Check sheet for the modelled part. Datum: model origin and axes. Units: mm. A direction names the side the tool comes from. Give positions to 0.01 mm unless a question says otherwise; leave off trailing zeros. Write each loop counter-clockwise with the first axis right and the second up, starting at its lowest first coordinate (ties: lowest second). Pieces come first, ordered by that corner, then holes. Notation, with made-up numbers: (-4, -16.5) - (5, -16.5) arc R12 cw to (5, 0.5) - close; hole circle Ø7 at (16, 82.25). An arc over 180 degrees is marked (long way). Return JSON: item names as keys, results as strings. Group by question number.
```python
from build123d import *

# Parameters (mm, degrees)
SKETCH_1_R           = 29
EXTRUDE_1_DEPTH      = 15
SKETCH_2_R           = 1.55
SKETCH_2_R_2         = 5.1
CUT_EXTRUDE_1_DEPTH  = 44.669211122
EXTRUDE_2_DEPTH      = 71
SKETCH_12_W          = 70
SKETCH_12_H          = 15
EXTRUDE_3_DEPTH      = 71
FILLET_5_R           = 10
SKETCH_22_W          = 71
SKETCH_22_H          = 103
CUT_EXTRUDE_11_DEPTH = 10
SKETCH_4_R           = 40
CUT_EXTRUDE_2_DEPTH  = 56
SKETCH_5_R           = 15.6
SKETCH_5_R_2         = 1.55
CUT_EXTRUDE_3_DEPTH  = 171.241005636
SKETCH_6_W           = 32.2
SKETCH_6_H           = 32.2
CUT_EXTRUDE_4_DEPTH  = 23.7
CUT_EXTRUDE_5_DEPTH  = 171.241005636
SKETCH_8_W           = 10
SKETCH_8_H           = 50
CUT_EXTRUDE_6_DEPTH  = 10
FILLET_1_R           = 10
FILLET_2_R           = 10
FILLET_3_R           = 10
SKETCH_17_R          = 22.5
CUT_EXTRUDE_7_DEPTH  = 7
SKETCH_18_R          = 24
CUT_EXTRUDE_8_DEPTH  = 0.5
EXTRUDE_START        = 10
SKETCH_19_R          = 15
SKETCH_19_R_2        = 1.55
SKETCH_19_R_3        = 5.1
EXTRUDE_5_DEPTH      = 10
SKETCH_20_R          = 3
CUT_EXTRUDE_9_DEPTH  = 3
SKETCH_23_R          = 1.5
CUT_EXTRUDE_12_DEPTH = 161.262160225
SKETCH_27_R          = 3
CUT_EXTRUDE_14_DEPTH = 3
SKETCH_28_W          = 10
SKETCH_28_H          = 6
EXTRUDE_6_DEPTH      = 5
FILLET_6_R           = 5
EXTRUDE_7_DEPTH      = 10
EXTRUDE_8_DEPTH      = 6


# Some blends are built 0.0001 mm under size
with BuildPart() as part:
    # Sketch 1 → Extrude 1 (new body)
    with BuildSketch(Plane.XY):
        Circle(SKETCH_1_R)
    extrude(amount=EXTRUDE_1_DEPTH)

    # Sketch 2 → Cut-Extrude 1 (cut, through all)
    with BuildSketch(Plane.XY.offset(15)):
        with Locations((-5.125, 8.876760389)):
            Circle(SKETCH_2_R)
        with Locations((5.125, 8.876760389)):
            Circle(SKETCH_2_R)
        with Locations((10.25, 0)):
            Circle(SKETCH_2_R)
        with Locations((5.125, -8.876760389)):
            Circle(SKETCH_2_R)
        Circle(SKETCH_2_R_2)
        with Locations((-5.125, -8.876760389)):
            Circle(SKETCH_2_R)
        with Locations((-10.25, 0)):
            Circle(SKETCH_2_R)
    extrude(amount=-CUT_EXTRUDE_1_DEPTH, mode=Mode.SUBTRACT)

    # Sketch 17 → Cut-Extrude 7 (cut)
    with BuildSketch(Plane.XY.offset(15)):
        Circle(SKETCH_17_R)
    extrude(amount=-CUT_EXTRUDE_7_DEPTH, mode=Mode.SUBTRACT)

    # Sketch 18 → Cut-Extrude 8 (cut)
    with BuildSketch(Plane.XY.offset(8)):
        Circle(SKETCH_18_R)
    extrude(amount=-CUT_EXTRUDE_8_DEPTH, mode=Mode.SUBTRACT)


with BuildPart() as body_2:
    # Sketch 3 → Extrude 2 (new body)
    with BuildSketch(Plane.XY):
        with BuildLine():
            ThreePointArc((-29, 0), (0, 29), (29, 0))
            Line((29, 0), (29, 95))
            Line((29, 95), (-9, 95))
            Line((-9, 95), (-9, 145))
            Line((-9, 145), (-29, 145))
            Line((-29, 145), (-29, 0))
        make_face()
    extrude(amount=EXTRUDE_2_DEPTH)

    # Sketch 12 → Extrude 3 (add)
    with BuildSketch(Plane.XY.offset(71)):
        with Locations((0, 34.5)):
            Rectangle(SKETCH_12_W, SKETCH_12_H)
    extrude(amount=-EXTRUDE_3_DEPTH)

    # Fillet 5
    # the kernel refuses this fillet: 10 mm, written as the material it takes off along each edge
    with BuildSketch(Plane(origin=(35, 42, 93.912878475), x_dir=(0, -1, 0), z_dir=(0, 0, -1))) as fillet_5_piece_1:
        with BuildLine():
            CenterArc((9.16515139, 10), FILLET_5_R, 203.578178478, 66.421821522)
            Line((0, 6), (-0.183303028, 5.92))
            ThreePointArc((-0.183303028, 5.92), (-0.2, 3), (-0.2, 0))
            Line((-0.2, 0), (0, -0.2))
            Line((0, -0.2), (9.16515139, -0.2))
            Line((9.16515139, -0.2), (9.16515139, 0))
        make_face()
    extrude(amount=116.82575695, mode=Mode.SUBTRACT)
    with BuildSketch(Plane(origin=(-35, 42, 93.912878475), x_dir=(0, -1, 0), z_dir=(0, 0, -1))) as fillet_5_piece_2:
        with BuildLine():
            CenterArc((9.16515139, -10), FILLET_5_R, 90, 66.421821522)
            Line((0, -6), (-0.183303028, -5.92))
            ThreePointArc((-0.183303028, -5.92), (-0.2, -3), (-0.2, 0))
            Line((-0.2, 0), (0, 0.2))
            Line((0, 0.2), (9.16515139, 0.2))
            Line((9.16515139, 0.2), (9.16515139, 0))
        make_face()
    extrude(amount=116.82575695, mode=Mode.SUBTRACT)

    # Sketch 22 → Cut-Extrude 11 (cut)
    with BuildSketch(Plane.ZY.offset(29)):
        with Locations((35.5, 93.5)):
            Rectangle(SKETCH_22_W, SKETCH_22_H)
    extrude(amount=-CUT_EXTRUDE_11_DEPTH, mode=Mode.SUBTRACT)

    # Sketch 4 → Cut-Extrude 2 (cut)
    with BuildSketch(Plane.XY.offset(71)):
        Circle(SKETCH_4_R)
    extrude(amount=-CUT_EXTRUDE_2_DEPTH, mode=Mode.SUBTRACT)

    # Sketch 5 → Cut-Extrude 3 (cut, through all)
    with BuildSketch(Plane.ZY.offset(19)):
        with Locations(Location((42.5, 70, 0), (0, 0, 270))):
            Circle(SKETCH_5_R)
        with Locations(Location((29.241747853, 83.258252147, 0), (0, 0, 270))):
            Circle(SKETCH_5_R_2)
        with Locations(Location((55.758252147, 83.258252147, 0), (0, 0, 270))):
            Circle(SKETCH_5_R_2)
        with Locations(Location((55.758252147, 56.741747853, 0), (0, 0, 270))):
            Circle(SKETCH_5_R_2)
        with Locations(Location((29.241747853, 56.741747853, 0), (0, 0, 270))):
            Circle(SKETCH_5_R_2)
    extrude(amount=-CUT_EXTRUDE_3_DEPTH, mode=Mode.SUBTRACT)

    # Sketch 6 → Cut-Extrude 4 (cut)
    with BuildSketch(Plane.ZY.offset(19)):
        with Locations((42.5, 70)):
            Rectangle(SKETCH_6_W, SKETCH_6_H)
    extrude(amount=-CUT_EXTRUDE_4_DEPTH, mode=Mode.SUBTRACT)

    # Sketch 7 → Cut-Extrude 5 (cut, through all)
    with BuildSketch(Plane.ZY.offset(19)):
        with BuildLine():
            Line((56.95, 137.497499937), (56.95, 133.497499937))
            ThreePointArc((56.95, 133.497499937), (58.5, 131.947499937), (60.05, 133.497499937))
            Line((60.05, 133.497499937), (60.05, 137.497499937))
            ThreePointArc((60.05, 137.497499937), (58.5, 139.047499937), (56.95, 137.497499937))
        make_face()
        with BuildLine():
            Line((54.1, 121.997499937), (54.1, 117.997499937))
            ThreePointArc((54.1, 117.997499937), (43, 106.897499937), (31.9, 117.997499937))
            Line((31.9, 117.997499937), (31.9, 121.997499937))
            ThreePointArc((31.9, 121.997499937), (43, 133.097499937), (54.1, 121.997499937))
        make_face()
        with BuildLine():
            Line((29.05, 137.497499937), (29.05, 133.497499937))
            ThreePointArc((29.05, 133.497499937), (27.5, 131.947499937), (25.95, 133.497499937))
            Line((25.95, 133.497499937), (25.95, 137.497499937))
            ThreePointArc((25.95, 137.497499937), (27.5, 139.047499937), (29.05, 137.497499937))
        make_face()
        with BuildLine():
            Line((56.95, 106.497499937), (56.95, 102.497499937))
            ThreePointArc((56.95, 102.497499937), (58.5, 100.947499937), (60.05, 102.497499937))
            Line((60.05, 102.497499937), (60.05, 106.497499937))
            ThreePointArc((60.05, 106.497499937), (58.5, 108.047499937), (56.95, 106.497499937))
        make_face()
        with BuildLine():
            Line((25.95, 106.497499937), (25.95, 102.497499937))
            ThreePointArc((25.95, 102.497499937), (27.5, 100.947499937), (29.05, 102.497499937))
            Line((29.05, 102.497499937), (29.05, 106.497499937))
            ThreePointArc((29.05, 106.497499937), (27.5, 108.047499937), (25.95, 106.497499937))
        make_face()
    extrude(amount=-CUT_EXTRUDE_5_DEPTH, mode=Mode.SUBTRACT)

    # Sketch 8 → Cut-Extrude 6 (cut)
    with BuildSketch(Plane(origin=(0, 0, 0), x_dir=(-1, 0, 0), z_dir=(0, 0, -1))):
        with Locations((14, 120)):
            Rectangle(SKETCH_8_W, SKETCH_8_H)
    extrude(amount=-CUT_EXTRUDE_6_DEPTH, mode=Mode.SUBTRACT)

    # Fillet 1
    fillet_1_edges = [body_2.edges().sort_by_distance(p)[0] for p in [
        (5, 95, 0),
    ]]
    fillet(fillet_1_edges, radius=FILLET_1_R)

    # Fillet 2
    fillet_2_edges = [body_2.edges().sort_by_distance(p)[0] for p in [
        (-14, 145, 10),
    ]]
    fillet(fillet_2_edges, radius=FILLET_2_R)

    # Fillet 3
    fillet_3_edges = [body_2.edges().sort_by_distance(p)[0] for p in [
        (-14, 145, 71),
    ]]
    fillet(fillet_3_edges, radius=FILLET_3_R)


    add(part.part)  # Extrude 5 merges part
    # Sketch 19 → Extrude 5 (add)
    with BuildSketch(Plane.XY.offset(7.5).offset(EXTRUDE_START)):
        Circle(SKETCH_19_R)
        with Locations((-5.125, -8.876760389)):
            Circle(SKETCH_19_R_2, mode=Mode.SUBTRACT)
        with Locations((5.125, -8.876760389)):
            Circle(SKETCH_19_R_2, mode=Mode.SUBTRACT)
        with Locations((10.25, 0)):
            Circle(SKETCH_19_R_2, mode=Mode.SUBTRACT)
        Circle(SKETCH_19_R_3, mode=Mode.SUBTRACT)
        with Locations((5.125, 8.876760389)):
            Circle(SKETCH_19_R_2, mode=Mode.SUBTRACT)
        with Locations((-5.125, 8.876760389)):
            Circle(SKETCH_19_R_2, mode=Mode.SUBTRACT)
        with Locations((-10.25, 0)):
            Circle(SKETCH_19_R_2, mode=Mode.SUBTRACT)
    extrude(amount=-EXTRUDE_5_DEPTH)

    # Sketch 20 → Cut-Extrude 9 (cut)
    with BuildSketch(Plane(origin=(0, 0, 0), x_dir=(-1, 0, 0), z_dir=(0, 0, -1))):
        with Locations((-5.125, 8.876760389)):
            Circle(SKETCH_20_R)
        with Locations((5.125, 8.876760389)):
            Circle(SKETCH_20_R)
        with Locations((-10.25, 0)):
            Circle(SKETCH_20_R)
        with Locations((-5.125, -8.876760389)):
            Circle(SKETCH_20_R)
        with Locations((5.125, -8.876760389)):
            Circle(SKETCH_20_R)
        with Locations((10.25, 0)):
            Circle(SKETCH_20_R)
    extrude(amount=-CUT_EXTRUDE_9_DEPTH, mode=Mode.SUBTRACT)

    # Sketch 23 → Cut-Extrude 12 (cut, through all)
    with BuildSketch(Plane(origin=(0, 0, 58.6), x_dir=(-1, 0, 0), z_dir=(0, 0, -1))):
        with Locations((-16, 80)):
            Circle(SKETCH_23_R)
        with Locations((9, 80)):
            Circle(SKETCH_23_R)
        with Locations((9, 55)):
            Circle(SKETCH_23_R)
        with Locations((-16, 55)):
            Circle(SKETCH_23_R)
    extrude(amount=-CUT_EXTRUDE_12_DEPTH, mode=Mode.SUBTRACT)

    # Sketch 27 → Cut-Extrude 14 (cut)
    with BuildSketch(Plane(origin=(29, 0, 0), x_dir=(0, 0, -1), z_dir=(1, 0, 0))):
        with Locations((-55.758252147, 83.258252147)):
            Circle(SKETCH_27_R)
        with Locations((-29.241747853, 83.258252147)):
            Circle(SKETCH_27_R)
        with Locations((-55.758252147, 56.741747853)):
            Circle(SKETCH_27_R)
        with Locations((-29.241747853, 56.741747853)):
            Circle(SKETCH_27_R)
    extrude(amount=-CUT_EXTRUDE_14_DEPTH, mode=Mode.SUBTRACT)

    # Sketch 28 → Extrude 6 (add)
    with BuildSketch(Plane(origin=(29, 0, 0), x_dir=(0, 0, -1), z_dir=(1, 0, 0))):
        with Locations((-63.1, 67)):
            Rectangle(SKETCH_28_W, SKETCH_28_H)
    extrude(amount=EXTRUDE_6_DEPTH)

    # Fillet 6
    fillet_6_edges = [body_2.edges().sort_by_distance(p)[0] for p in [
        (29, 64, 63.1),
    ]]
    fillet(fillet_6_edges, radius=FILLET_6_R - 0.0001)  # a hair under: the kernel refuses the full size

    # Sketch 29 → Extrude 7 (add)
    with BuildSketch(Plane(origin=(0, 0, 0), x_dir=(-1, 0, 0), z_dir=(0, 0, -1))):
        Polygon((19, 70), (29, 42), (19, 42), align=None)
    extrude(amount=-EXTRUDE_7_DEPTH)

    # Sketch 30 → Extrude 8 (add)
    with BuildSketch(Plane.XY.offset(71)):
        Polygon((-29, 42), (-19, 70), (-19, 42), align=None)
    extrude(amount=-EXTRUDE_8_DEPTH)


solid = body_2.part
```
Item 1: Section check A-A on x = 0. Record the cut outline in (y, z), plus the area to 3 significant figures.
Item 2: Material ranges on line 1 along Y through (x, z) = (13, 29); line 2 along X through (y, z) = (82, 28); line 3 along X through (y, z) = (92.5, 39.5), recorded low to high. Write a range as from..to.
Item 3: Depth check by flat-ended pin: pin 1 (1.5 mm diameter, centred on x = 22, z = 24.5, fed in from -Y); pin 2 (4 mm diameter, centred on x = 20.5, z = 59.5, fed in from +Y); pin 3 (5.5 mm diameter, centred on x = 32, y = 66, fed in from +Z). Enter the tip coordinate at first touch or a pass-through.
Item 4: Section check B-B on z = 51. Record the cut outline in (x, y).
Item 5: Mould release check, pull along X, two halves, no side actions. Record for faces 6 (the face through (9.02, -0.94, 10.35)), 7 (the face through (27.521, 84.159, 52.897)), 8 (the face through (-6.27, -7.83, 10.35)), 9 (the face through (33.32, 38.38, 36)): +X half, -X half, draft (parallel to the pull), parting line (faces both ways), or undercut.
Item 6: Access from +Z, -Z, +X, -X, +Y, -Y to the whole of each face (thin tool, end or side, straight path). Record for faces 1 (the face through (-14.07, 133.095, 42.756)), 2 (the face through (6, 0, 17.5)), 3 (the face through (-14.985, 0.66, 12.57)), 4 (the face through (-14, 115, 10)), 5 (the face through (27.52, 55.59, 26.47)).
Item 7: Section check C-C on z = 42.5. Record the cut outline in (x, y), plus the area to 3 significant figures.
Reply:
{
 "1": {"outline": "(-29, 0) - (-5.1, 0) - (-5.1, 17.5) - (-15, 17.5) - (-15, 7.5) - (-24, 7.5) - (-24, 8) - (-22.5, 8) - (-22.5, 15) - (-29, 15) - close; (5.1, 0) - (85, 0) arc R10 ccw to (95, 10) - (95, 71) - (40, 71) - (40, 15) - (22.5, 15) - (22.5, 8) - (24, 8) - (24, 7.5) - (15, 7.5) - (15, 17.5) - (5.1, 17.5) - close; hole (53.9, 26.4) - (86.1, 26.4) - (86.1, 58.6) - (53.9, 58.6) - close", "area": "3,660 mm²"},
 "2": {"line 1": "37.83..55.21, 58.27..62.18, 77.82..81.73, 84.79..95", "line 2": "4.7..26", "line 3": "-19..29"},
 "3": {"pin 1": "y = 32.9", "pin 2": "y = 95", "pin 3": "z = 68.1"},
 "4": {"outline": "(-35, 27) - (-29.51, 27) arc R40 cw to (29.51, 27) - (35, 27) - (35, 32.83) arc R10 ccw to (29, 42) - (29, 56.92) - (4.7, 56.92) - (4.7, 53.9) - (-19, 53.9) - (-19, 42) - (-29, 42) arc R10 ccw to (-35, 32.83) - close; (-19, 86.1) - (4.7, 86.1) - (4.7, 83.08) - (29, 83.08) - (29, 95) - (-9, 95) - (-9, 110.3) - (-19, 110.3) - close; (-19, 129.69) - (-9, 129.69) - (-9, 145) - (-19, 145) - close"},
 "5": {"face 6": "undercut", "face 7": "draft", "face 8": "undercut", "face 9": "+X half"},
 "6": {"face 1": "+X, -X", "face 2": "+Z, +X, -X, -Y", "face 3": "+Z", "face 4": "-Z, +X, -X, +Y", "face 5": "+X"},
 "7": {"outline": "(-35, 27) - (-29.51, 27) arc R40 cw to (29.51, 27) - (35, 27) - (35, 32.83) arc R10 ccw to (29, 42) - (29, 54.4) - (4.7, 54.4) - (4.7, 53.9) - (-19, 53.9) - (-19, 42) - (-29, 42) arc R10 ccw to (-35, 32.83) - close; (-19, 86.1) - (4.7, 86.1) - (4.7, 85.6) - (29, 85.6) - (29, 95) - (-9, 95) - (-9, 106.91) - (-19, 106.91) - close; (-19, 133.09) - (-9, 133.09) - (-9, 145) - (-19, 145) - close", "area": "1,750 mm²"}
}
